For this review, take the finished solid that the model builds, in its own axes (mm). Face numbers are marked on the shaded views. A direction names the side the tool comes from. Coordinates: 2 decimals unless noted, no trailing zeros. Write each loop counter-clockwise with the first axis right and the second up, starting at its lowest first coordinate (ties: lowest second). Pieces come first, ordered by that corner, then holes. Notation, with made-up numbers: (11.25, 32.5) - (62.25, 32.5) arc R24 ccw to (62.25, 70.5) - close; hole circle Ø9 at (6, 61.5). An arc over 180 degrees is marked (long way). Use one line per item in the form item = value. Start each with the question number.
1) For L1, parallel to Z at x = -39.5, y = 18.5; L2, parallel to Z at x = -30, y = -32.5; L3, parallel to X at y = -40.5, z = 80, list the stretches that pass through material, from the lowest coordinate up. Write a range as from..to.
2) We need section A-A (z = 65.5). Give the boundary of the cut face in (x, y).
3) Mouldability with a two-part tool opening along X and no side actions: class the marked faces 1, 2 and 3 as pulls with the +X half, pulls with the -X half, needs draft (parallel to the pull), parting line crosses it, or undercut.
4) Insertion check: P1, Ø3, axis at x = 50, z = -7.5, coming from the -Y side; P2, Ø1.5, axis at y = 3, z = 13.5, coming from the -X side; P3, Ø8, axis at x = 15, y = 56, coming from the -Z side. Each pin has a flat end and moves straight along its axis. Give the tip position at first contact, or say it passes through.
5) Tool access review of the marked faces 4, 5 and 6: name each direction out of +Z, -Z, +X, -X, +Y, -Y from which nothing blocks a thin tool from reaching the whole face with its end or side.
```python
from build123d import *

# Parameters (mm, degrees)
F0_R     = 70.4060521859
F1_DEPTH = 45.212
F1_TAPER = -3
F4_DEPTH = 25.4
F6_DEPTH = 76.2


with BuildPart() as f1:
    # F0 (on Top) → F1 (new body)
    with BuildSketch(Plane.XY):
        Circle(F0_R)
    extrude(amount=F1_DEPTH, taper=F1_TAPER)

    # F3 (on face) → F4 (join)
    with BuildSketch(Plane.XY):
        Polygon((13.2651496679, 8.6820758879), (22.1880245954, 8.6820758879), (20.0088638812, 20.2589873224), align=None)
        Polygon((26.7175994813, 37.1265895665), (39.3666066229, 41.3835719228), (26.7175994813, 50.9552955627), align=None)
        Polygon((0, 41.3835719228), (0, 62.2292943299), (-9.2889685184, 54.0895685554), align=None)
        Polygon((-17.2152053565, 4.2226207443), (-10.1358499378, 0), (-11.7327948169, 13.4140530589), align=None)
        Polygon((-12.0866000652, -31.0505852103), (-4.3377871625, -31.0505852103), (-10.1358499378, -17.055625096), align=None)
        Polygon((0, -59.9799224224), (12.0000867173, -55.9413321316), (0, -43.2448089123), align=None)
        Polygon((45.8979159594, 8.6820758879), (58.5819035769, 4.2226207443), (50.1223825414, 20.6976876816), align=None)
        Polygon((-40.3976216912, 35.750195384), (-30.278051272, 30.9688523412), (-35.5101494777, 46.0943850381), align=None)
        Polygon((-52.9398620129, -27.6039075106), (-45.7244627178, -17.1867813915), (-56.9789598161, -15.6023127936), align=None)
        Polygon((8.7098376591, -20.6725607113), (19.0673265606, -17.1867813915), (12.0000867173, -7.1116369218), align=None)
        Polygon((-38.8014949858, 4.2226207443), (-30.278051272, 4.2226207443), (-34.1327454541, 15.676286782), align=None)
        Polygon((-41.7802073061, -50.3433160484), (-32.6245762408, -50.3433160484), (-34.0931266546, -39.8950539529), align=None)
        Polygon((43.1729927659, 30.9688523412), (53.0351176858, 30.9688523412), (45.9125488997, 45.8067990839), align=None)
    extrude(amount=-F4_DEPTH)

    # F5 (on face) → F6 (join)
    with BuildSketch(Plane.XY.offset(45.212)):
        with BuildLine():
            Line((-2.7060096618, -60.9949491918), (15.9434843808, -17.7769623697))
            ThreePointArc((15.9434843808, -17.7769623697), (-43.1665021025, -17.9025504898), (-2.7060096618, -60.9949491918))
        make_face()
    extrude(amount=F6_DEPTH)


solid = f1.part
```
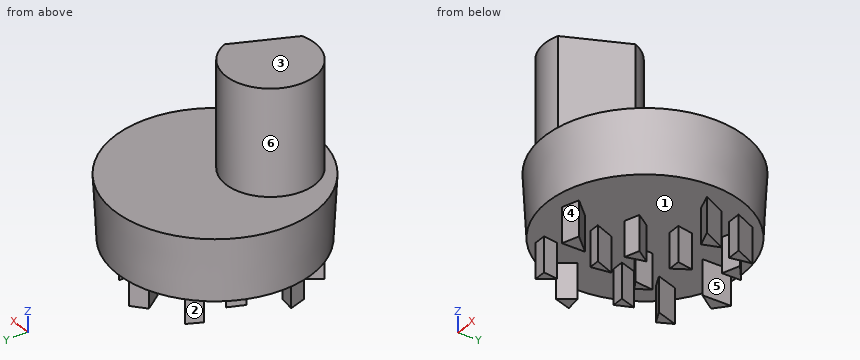
Determined:
q1.L1 = 0..45.21
q1.L2 = 0..121.41
q1.L3 = -44.27..6.14
q2.outline = (-2.71, -60.99) - (15.94, -17.78) arc R32.22 ccw (long way) to start
q3.face_1 = undercut
q3.face_2 = pulls with the -X half
q3.face_3 = needs draft
q4.P1 = 6.71
q4.P2 = -71.1
q4.P3 = 0
q5.face_4 = -Z, +X, -Y
q5.face_5 = -Z, +Y
q5.face_6 = +Z
